from build123d import *

# Parameters (mm, degrees)
BOSS_EXTRUDE1_DEPTH = 6.35
SKETCH9_R           = 1.65
CUT_EXTRUDE10_DEPTH = 30
CUT_EXTRUDE12_DEPTH = 30
SKETCH10_R          = 1.65
CUT_EXTRUDE13_DEPTH = 10
SKETCH12_R          = 35
CUT_EXTRUDE14_DEPTH = 192.836707905
SKETCH13_R          = 2.25
CUT_EXTRUDE15_DEPTH = 192.836707905
SKETCH14_R          = 25
CUT_EXTRUDE16_DEPTH = 10
SKETCH15_R          = 1.175
CUT_EXTRUDE17_DEPTH = 10


with BuildPart() as part:
    # Sketch1 → Boss-Extrude1 (new body)
    with BuildSketch(Plane(origin=(0, 0, 0), x_dir=(1, 0, 0), z_dir=(0, 1, 0))):
        Polygon((-71, 140), (71, 140), (71, -140), (-131, -140), (-131, 120), (-71, 120), align=None)
    extrude(amount=BOSS_EXTRUDE1_DEPTH)

    # Sketch9 → Cut-Extrude10 (cut)
    with BuildSketch(Plane(origin=(0, 0, 0), x_dir=(-1, 0, 0), z_dir=(0, -1, 0))):
        with Locations(Location((45.6, 129.325, 0), (0, 0, 90))):
            Circle(SKETCH9_R)
        with Locations(Location((5.6, 129.325, 0), (0, 0, 90))):
            Circle(SKETCH9_R)
        with Locations(Location((-34.4, 129.325, 0), (0, 0, 90))):
            Circle(SKETCH9_R)
        with Locations(Location((65.6, 129.325, 0), (0, 0, 90))):
            Circle(SKETCH9_R)
        with Locations(Location((25.6, 129.325, 0), (0, 0, 90))):
            Circle(SKETCH9_R)
        with Locations(Location((-14.4, 129.325, 0), (0, 0, 90))):
            Circle(SKETCH9_R)
        with Locations(Location((-54.4, 129.325, 0), (0, 0, 90))):
            Circle(SKETCH9_R)
    extrude(amount=-CUT_EXTRUDE10_DEPTH, mode=Mode.SUBTRACT)

    # Sketch11 → Cut-Extrude12 (cut)
    with BuildSketch(Plane(origin=(0, 6.35, 0), x_dir=(1, 0, 0), z_dir=(0, 1, 0))):
        with BuildLine():
            Line((-63.95, -128.355), (-63.95, -131.655))
            ThreePointArc((-63.95, -131.655), (-65.6, -133.305), (-67.25, -131.655))
            Line((-67.25, -131.655), (-67.25, -128.355))
            ThreePointArc((-67.25, -128.355), (-65.6, -126.705), (-63.95, -128.355))
        make_face()
        with BuildLine():
            Line((-23.95, -128.353535871), (-23.95, -131.653535871))
            ThreePointArc((-23.95, -131.653535871), (-25.6, -133.303535871), (-27.25, -131.653535871))
            Line((-27.25, -131.653535871), (-27.25, -128.353535871))
            ThreePointArc((-27.25, -128.353535871), (-25.6, -126.703535871), (-23.95, -128.353535871))
        make_face()
        with BuildLine():
            Line((16.05, -128.352071742), (16.05, -131.652071742))
            ThreePointArc((16.05, -131.652071742), (14.4, -133.302071742), (12.75, -131.652071742))
            Line((12.75, -131.652071742), (12.75, -128.352071742))
            ThreePointArc((12.75, -128.352071742), (14.4, -126.702071742), (16.05, -128.352071742))
        make_face()
        with BuildLine():
            Line((56.05, -128.350607613), (56.05, -131.650607613))
            ThreePointArc((56.05, -131.650607613), (54.4, -133.300607613), (52.75, -131.650607613))
            Line((52.75, -131.650607613), (52.75, -128.350607613))
            ThreePointArc((52.75, -128.350607613), (54.4, -126.700607613), (56.05, -128.350607613))
        make_face()
    extrude(amount=-CUT_EXTRUDE12_DEPTH, mode=Mode.SUBTRACT)

    # Sketch10 → Cut-Extrude13 (cut)
    with BuildSketch(Plane.XZ):
        with Locations((-120.325, -110)):
            Circle(SKETCH10_R)
        with BuildLine():
            Line((-118.675, -108.35), (-120.325, -108.35))
            ThreePointArc((-120.325, -108.35), (-119.158273811, -108.833273811), (-118.675, -110))
            ThreePointArc((-118.675, -110), (-119.158273801, -111.166726179), (-120.324999972, -111.65))
            Line((-120.324999972, -111.65), (-118.675, -111.65))
            ThreePointArc((-118.675, -111.65), (-117.025, -110), (-118.675, -108.35))
        make_face()
        with BuildLine():
            Line((-120.325, -108.35), (-121.975, -108.35))
            ThreePointArc((-121.975, -108.35), (-123.625, -110), (-121.975, -111.65))
            Line((-121.975, -111.65), (-120.324999972, -111.65))
            ThreePointArc((-120.324999972, -111.65), (-121.975, -110.000000014), (-120.325, -108.35))
        make_face()
        with BuildLine():
            Line((-120.325, -48.35), (-121.975, -48.35))
            ThreePointArc((-121.975, -48.35), (-123.625, -50), (-121.975, -51.65))
            Line((-121.975, -51.65), (-120.325, -51.65))
            ThreePointArc((-120.325, -51.65), (-121.975, -50), (-120.325, -48.35))
        make_face()
        with Locations((-120.325, -50)):
            Circle(SKETCH10_R)
        with BuildLine():
            Line((-118.675, -48.35), (-120.325, -48.35))
            ThreePointArc((-120.325, -48.35), (-119.158273811, -48.833273811), (-118.675, -50))
            ThreePointArc((-118.675, -50), (-119.158273811, -51.166726189), (-120.325, -51.65))
            Line((-120.325, -51.65), (-118.675, -51.65))
            ThreePointArc((-118.675, -51.65), (-117.025, -50), (-118.675, -48.35))
        make_face()
        with BuildLine():
            Line((-120.325, 11.65), (-121.975, 11.65))
            ThreePointArc((-121.975, 11.65), (-123.625, 10), (-121.975, 8.35))
            Line((-121.975, 8.35), (-120.325, 8.35))
            ThreePointArc((-120.325, 8.35), (-121.975, 10), (-120.325, 11.65))
        make_face()
        with Locations((-120.325, 10)):
            Circle(SKETCH10_R)
        with BuildLine():
            Line((-118.675, 11.65), (-120.325, 11.65))
            ThreePointArc((-120.325, 11.65), (-119.158273811, 11.166726189), (-118.675, 10))
            ThreePointArc((-118.675, 10), (-119.158273811, 8.833273811), (-120.325, 8.35))
            Line((-120.325, 8.35), (-118.675, 8.35))
            ThreePointArc((-118.675, 8.35), (-117.025, 10), (-118.675, 11.65))
        make_face()
        with BuildLine():
            Line((-120.325, 71.65), (-121.975, 71.65))
            ThreePointArc((-121.975, 71.65), (-123.625, 70), (-121.975, 68.35))
            Line((-121.975, 68.35), (-120.325, 68.35))
            ThreePointArc((-120.325, 68.35), (-121.975, 70), (-120.325, 71.65))
        make_face()
        with Locations((-120.325, 70)):
            Circle(SKETCH10_R)
        with BuildLine():
            Line((-118.675, 71.65), (-120.325, 71.65))
            ThreePointArc((-120.325, 71.65), (-119.158273811, 71.166726189), (-118.675, 70))
            ThreePointArc((-118.675, 70), (-119.158273811, 68.833273811), (-120.325, 68.35))
            Line((-120.325, 68.35), (-118.675, 68.35))
            ThreePointArc((-118.675, 68.35), (-117.025, 70), (-118.675, 71.65))
        make_face()
    extrude(amount=-CUT_EXTRUDE13_DEPTH, mode=Mode.SUBTRACT)

    # Sketch12 → Cut-Extrude14 (cut, through all)
    with BuildSketch(Plane(origin=(0, 6.35, 0), x_dir=(1, 0, 0), z_dir=(0, 1, 0))):
        with Locations(Location((-29, 60, 0), (0, 0, 270))):
            Circle(SKETCH12_R)
    extrude(amount=-CUT_EXTRUDE14_DEPTH, mode=Mode.SUBTRACT)

    # Sketch13 → Cut-Extrude15 (cut, through all)
    with BuildSketch(Plane(origin=(0, 6.35, 0), x_dir=(1, 0, 0), z_dir=(0, 1, 0))):
        with Locations(Location((-90.25, 60, 0), (0, 0, 270))):
            Circle(SKETCH13_R)
        with Locations(Location((-59.625, 113.044055982, 0), (0, 0, 270))):
            Circle(SKETCH13_R)
        with Locations(Location((1.625, 113.044055982, 0), (0, 0, 270))):
            Circle(SKETCH13_R)
        with Locations(Location((32.25, 60, 0), (0, 0, 270))):
            Circle(SKETCH13_R)
        with Locations(Location((1.625, 6.955944018, 0), (0, 0, 270))):
            Circle(SKETCH13_R)
        with Locations(Location((-59.625, 6.955944018, 0), (0, 0, 270))):
            Circle(SKETCH13_R)
    extrude(amount=-CUT_EXTRUDE15_DEPTH, mode=Mode.SUBTRACT)

    # Sketch14 → Cut-Extrude16 (cut)
    with BuildSketch(Plane(origin=(0, 6.35, 0), x_dir=(1, 0, 0), z_dir=(0, 1, 0))):
        with Locations(Location((-29, -70, 0), (0, 0, 270))):
            Circle(SKETCH14_R)
    extrude(amount=-CUT_EXTRUDE16_DEPTH, mode=Mode.SUBTRACT)

    # Sketch15 → Cut-Extrude17 (cut)
    with BuildSketch(Plane(origin=(0, 6.35, 0), x_dir=(1, 0, 0), z_dir=(0, 1, 0))):
        with Locations(Location((-111.024467158, 25.298909731, 0), (0, 0, 270))):
            Circle(SKETCH15_R)
        with Locations(Location((-106.983736963, 16.701090269, 0), (0, 0, 270))):
            Circle(SKETCH15_R)
    extrude(amount=-CUT_EXTRUDE17_DEPTH, mode=Mode.SUBTRACT)


solid = part.part
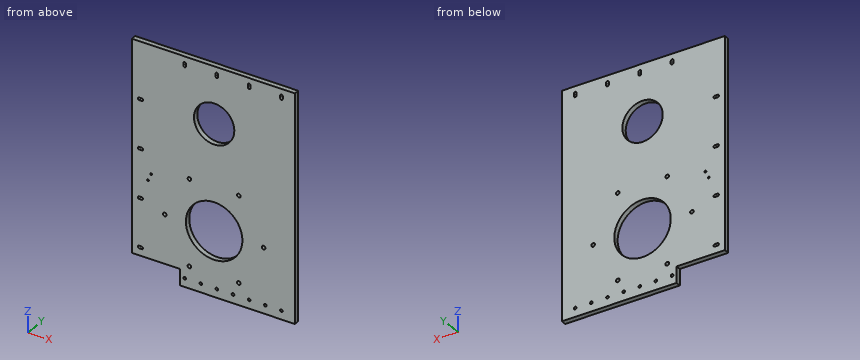
Check sheet for the modelled part. Datum: model origin and axes. Units: mm. Give positions to 0.01 mm unless a question says otherwise; leave off trailing zeros. Write each loop counter-clockwise with the first axis right and the second up, starting at its lowest first coordinate (ties: lowest second). Pieces come first, ordered by that corner, then holes. Notation, with made-up numbers: (17, 74) -> (27, 74) arc R13 cw to (27, 85) -> close; hole circle Ø11 at (14.5, -10). An arc over 180 degrees is marked (long way). Write item = value, one per line.
Item 1: Sectioned sample at A-A on z = 85. Record the boundary of the cut face in (x, y).
Output:
outline = (-131, 0) -> (-49, 0) -> (-49, 6.35) -> (-131, 6.35) -> close; (-9, 0) -> (71, 0) -> (71, 6.35) -> (-9, 6.35) -> close
Item 2: Sectioned sample at B-B on x = -20.5. Record the boundary of the cut face in (y, z).
Output:
outline = (0, -140) -> (6.35, -140) -> (6.35, -93.95) -> (0, -93.95) -> close; (0, -26.05) -> (6.35, -26.05) -> (6.35, 46.49) -> (0, 46.49) -> close; (0, 93.51) -> (6.35, 93.51) -> (6.35, 140) -> (0, 140) -> close
Item 3: Gauge pin test, flat ends, axial feed: pin 1 (6 mm diameter, centred on x = -81.5, z = -36, fed in from -Y); pin 2 (2.5 mm diameter, centred on x = -5.6, z = -129.325, fed in from +Y). Record the tip position at first contact, or that the pin passes through.
Output:
pin_1 = 0
pin_2 = through
Item 4: Sectioned sample at D-D on x = -76.5. Record the boundary of the cut face in (y, z), and give its area (3 significant figures).
Output:
outline = (0, -120) -> (6.35, -120) -> (6.35, 140) -> (0, 140) -> close
area = 1,650 mm^2
Item 5: Sectioned sample at C-C on y = 4.5. Count the separate pieces of the cut face and the enclosed holes in it, and give its area (3 significant figures).
Output:
separate_pieces = 1
enclosed_holes = 25
area = 49,200 mm^2
Item 6: Scan lines: probe 1 along Z at (x, y) = (-121, 0.75); probe 2 along Z at (x, y) = (-65.5, 4.25); probe 3 along X at (y, z) = (2, 70) (3 decimals). Record each from-to range of solid material in increasing order. Write a range as from..to.
Output:
probe_1 = -120..-111.65, -108.35..-51.65, -48.35..8.35, 11.65..68.35, 71.65..140
probe_2 = -140..-130.97, -127.68..126.71, 133.3..140
probe_3 = -131..-123.625, -117.025..-54, -4..71
